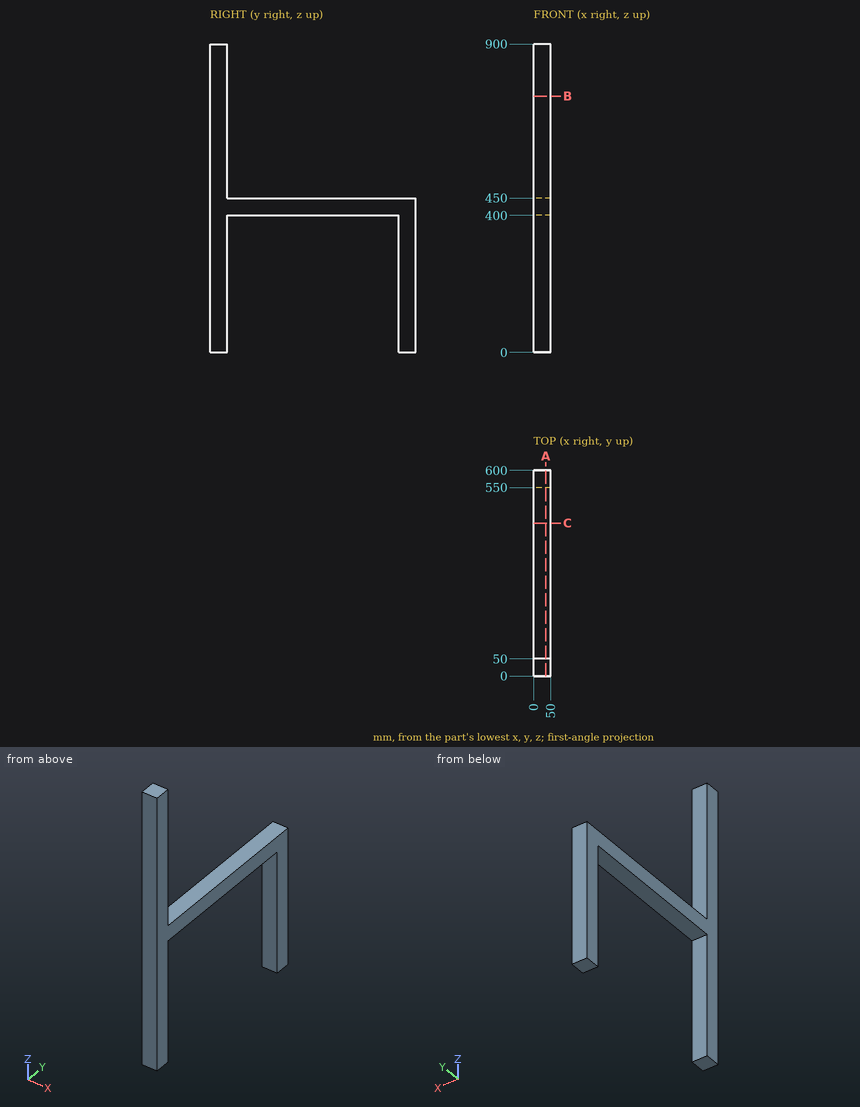
The figure shows three views and two pictorial views of one solid part (mm, origin at its lowest corner). Answer the questions. Coordinates: 2 decimals unless noted, no trailing zeros. Write each loop counter-clockwise with the first axis right and the second up, starting at its lowest first coordinate (ties: lowest second). Pieces come first, ordered by that corner, then holes. Notation, with made-up numbers: M -38.5,56 L -4.5,56 A30 ccw -4.5,87 Z; hole C -3,48 d10. An arc over 180 degrees is marked long. Answer as CSV lines item,"result". Start each with the question number.
Item 1: Consider L1, parallel to Y at x = 8, z = 151; L2, parallel to Z at x = 19, y = 147; L3, parallel to Y at x = 10, z = 751.5. Determine where each line is inside the solid, lowest interval first.
Item 2: Section B-B on z = 748 is taken. Write down the section's boundary in (x, y), and give its area (3 significant figures).
Item 3: Section C-C on y = 446 is taken. Write down the section's boundary in (x, z).
Item 4: Section A-A on x = 35.5 is taken. Write down the section's boundary in (y, z).
Item 5: Flat-ended cylindrical pins translate along their axes: P1, Ø5, axis at x = 27, z = 747.5, coming from the +Y side; P2, Ø6, axis at x = 33, y = 99, coming from the -Z side; P3, Ø6, axis at x = 23, y = 147, coming from the +Z side. Find the tip coordinate at first contact, or state that the pin passes through.
Checks:
1,L1,"y = 0 to 50, 550 to 600"
1,L2,"z = 400 to 450"
1,L3,"y = 0 to 50"
2,outline,"M 0,0 L 50,0 L 50,50 L 0,50 Z"
2,area,"2,500 mm²"
3,outline,"M 0,400 L 50,400 L 50,450 L 0,450 Z"
4,outline,"M 0,0 L 50,0 L 50,400 L 550,400 L 550,0 L 600,0 L 600,450 L 50,450 L 50,900 L 0,900 Z"
5,P1,"stops at y = 50"
5,P2,"stops at z = 400"
5,P3,"stops at z = 450"
